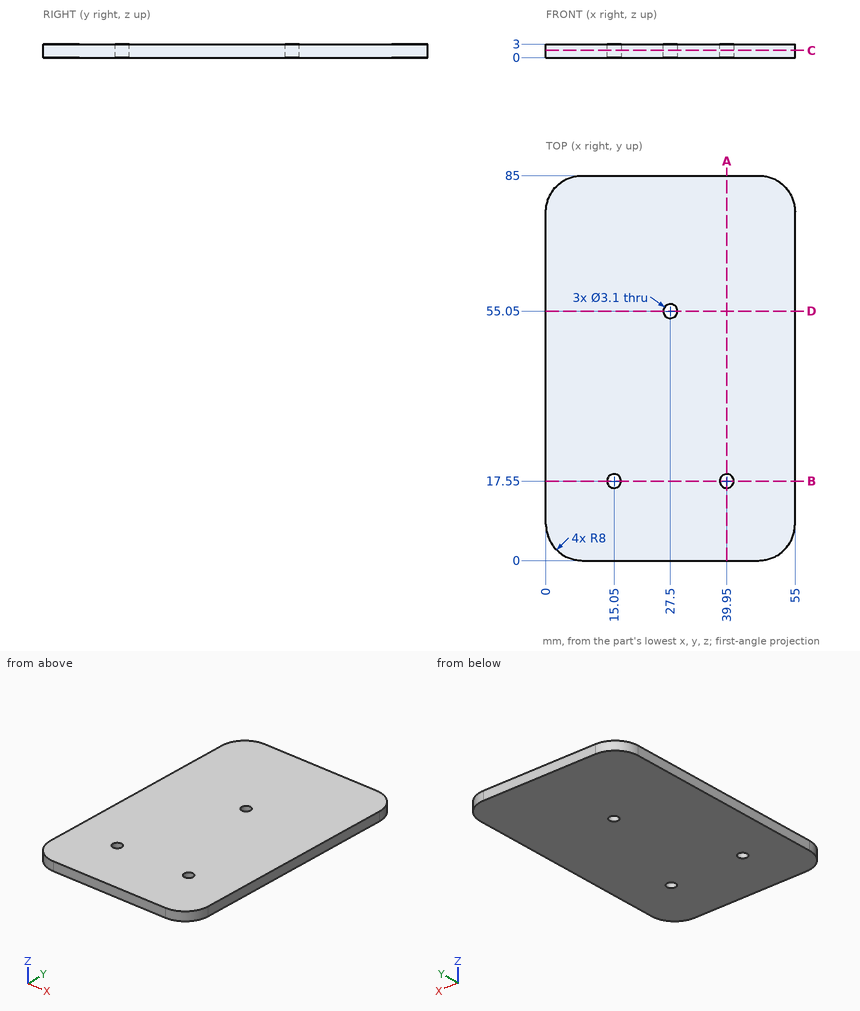
Study the drawing (mm; zero at the part's minimum x, y, z) and answer. Round coordinates to 2 decimals unless told otherwise and drop trailing zeros. Write each loop counter-clockwise with the first axis right and the second up, starting at its lowest first coordinate (ties: lowest second). Pieces come first, ordered by that corner, then holes. Notation, with made-up numbers: (-28.75, 26.5) - (-16.75, 26.5) arc R23 cw to (-16.75, 62.5) - close; hole circle Ø7 at (31.25, 48.25). An arc over 180 degrees is marked (long way). Return JSON: item names as keys, results as strings. Group by question number.
Q1. Find the intervals of material crossed by L1, parallel to Y at x = 15.05, z = 1.9; L2, parallel to Y at x = 27.5, z = 2.3; L3, parallel to Y at x = 4, z = 2.85, in increasing order.
Q2. The part is cut by section C-C on z = 1.6. Write down the section's boundary in (x, y).
Q3. The part is cut by section D-D on y = 55.05. Write down the section's boundary in (x, z).
Q4. The part is cut by section B-B on y = 17.55. Write down the section's boundary in (x, z), then the cut area to 3 significant figures.
Q5. The part is cut by section A-A on x = 39.95. Write down the section's boundary in (y, z).
Solved:
{
 "1": {"L1": "0 to 16, 19.1 to 85", "L2": "0 to 53.5, 56.6 to 85", "L3": "1.07 to 83.93"},
 "2": {"outline": "(0, 8) arc R8 ccw to (8, 0) - (47, 0) arc R8 ccw to (55, 8) - (55, 77) arc R8 ccw to (47, 85) - (8, 85) arc R8 ccw to (0, 77) - close; hole circle Ø3.1 at (15.05, 17.55); hole circle Ø3.1 at (27.5, 55.05); hole circle Ø3.1 at (39.95, 17.55)"},
 "3": {"outline": "(0, 0) - (25.95, 0) - (25.95, 3) - (0, 3) - close; (29.05, 0) - (55, 0) - (55, 3) - (29.05, 3) - close"},
 "4": {"outline": "(0, 0) - (13.5, 0) - (13.5, 3) - (0, 3) - close; (16.6, 0) - (38.4, 0) - (38.4, 3) - (16.6, 3) - close; (41.5, 0) - (55, 0) - (55, 3) - (41.5, 3) - close", "area": "146 mm²"},
 "5": {"outline": "(0, 0) - (16, 0) - (16, 3) - (0, 3) - close; (19.1, 0) - (85, 0) - (85, 3) - (19.1, 3) - close"}
}
